Source: three-view drawing plus pictorial views. Frame: mm from the lowest corner of the part. A direction names the side the tool comes from. Give positions to 0.01 mm unless a question says otherwise; leave off trailing zeros. Loops run counter-clockwise (first coordinate to the right, second up) from the corner with the lowest first, then second, coordinate; pieces in that order, holes last.
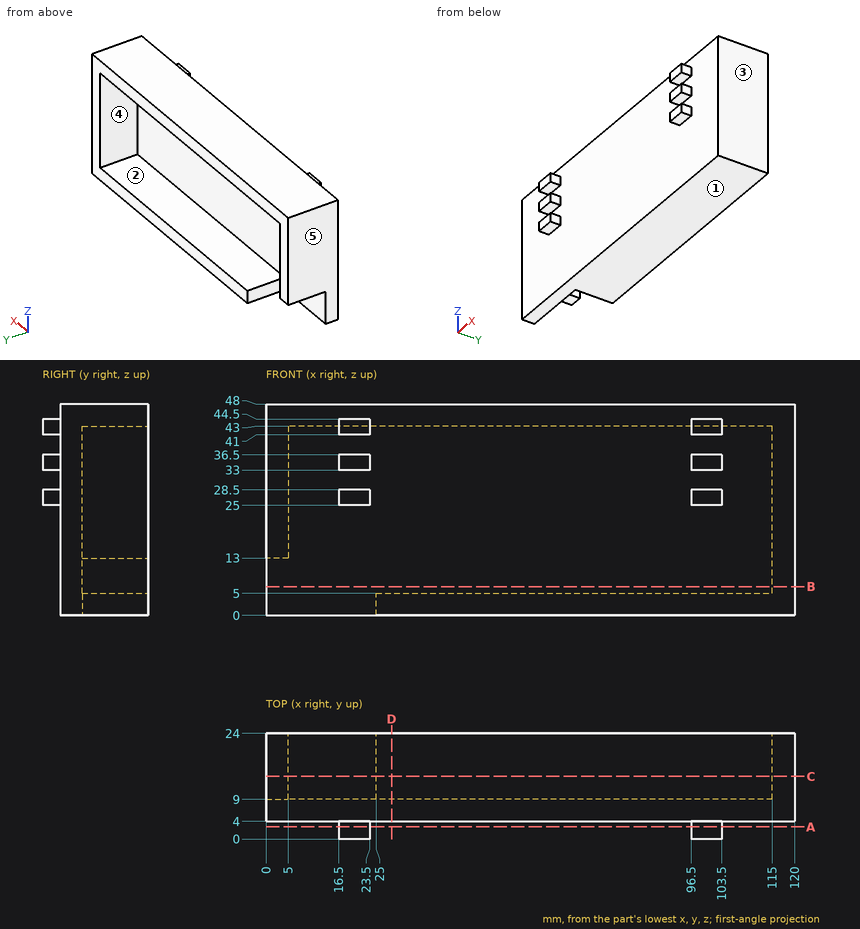
Q1. Section query A-A, the plane y = 2.75. Return loops of the section in (x, z), and give its area (3 significant figures).
Q2. Section query D-D, the plane x = 28.5. Return loops of the section in (y, z), and give its area (3 significant figures).
Q3. Section query B-B, the plane z = 6.5. Return loops of the section in (x, y), and give its area (3 significant figures).
Q4. Mould query, pull axis Z, two halves, no side actions, for the marked faces 1, 2 and 3. Classes: +Z half, -Z half, draft (parallel to the pull), parting line (faces both ways), or undercut.
Q5. Section query C-C, the plane y = 14.25. Return loops of the section in (x, z), and give its area (4 significant figures).
Q6. Material intervals for probe 1 along X at (y, z) = (17.5, 17); probe 2 along Z at (x, y) = (110, 21.25); probe 3 along X at (y, z) = (1, 26), sorted ascending.
Q7. Pin query (flat end, axial travel): pin 1 Ø2 at (x, y) = (99.5, 1) entering from -Z; pin 2 Ø1 at (x, y) = (72, 20) entering from -Z; pin 3 Ø1 at (y, z) = (1.5, 42) entering from +X; pin 4 Ø2 at (x, y) = (20.5, 2.5) entering from +Z. Return the tip coordinate at first contact, or that it passes through.
Q8. Reachability of the marked faces 4 and 5 from +Z, -Z, +X, -X, +Y, -Y: full face, straight path, thin tool, end or side. Return the list, or none.
Resolved:
1. outline: (16.5, 25) - (23.5, 25) - (23.5, 28.5) - (16.5, 28.5) - close; (16.5, 33) - (23.5, 33) - (23.5, 36.5) - (16.5, 36.5) - close; (16.5, 41) - (23.5, 41) - (23.5, 44.5) - (16.5, 44.5) - close; (96.5, 25) - (103.5, 25) - (103.5, 28.5) - (96.5, 28.5) - close; (96.5, 33) - (103.5, 33) - (103.5, 36.5) - (96.5, 36.5) - close; (96.5, 41) - (103.5, 41) - (103.5, 44.5) - (96.5, 44.5) - close
1. area: 147 mm2
2. outline: (4, 0) - (24, 0) - (24, 5) - (9, 5) - (9, 43) - (24, 43) - (24, 48) - (4, 48) - close
2. area: 390 mm2
3. outline: (0, 4) - (120, 4) - (120, 24) - (115, 24) - (115, 9) - (0, 9) - close
3. area: 675 mm2
4. face 1: -Z half
4. face 2: undercut
4. face 3: draft
5. outline: (0, 13) - (5, 13) - (5, 43) - (115, 43) - (115, 5) - (25, 5) - (25, 0) - (120, 0) - (120, 48) - (0, 48) - close
5. area: 1,415 mm2
6. probe 1: x = 0 to 5, 115 to 120
6. probe 2: z = 0 to 5, 43 to 48
6. probe 3: x = 16.5 to 23.5, 96.5 to 103.5
7. pin 1: stops at z = 25
7. pin 2: stops at z = 0
7. pin 3: stops at x = 103.5
7. pin 4: stops at z = 44.5
8. face 4: +Y
8. face 5: +Z, -Z, -X, +Y, -Y
